The figure shows three views and two pictorial views of one solid part (mm, origin at its lowest corner). Answer the questions. Coordinates: 2 decimals unless noted, no trailing zeros. Order: outer loops, then holes, each group sorted by start corner. A loop starts at its lowest first (then second) coordinate and runs counter-clockwise, first axis right, second up. Notation, with made-up numbers: (17.25, 25) -> (72.25, 25) arc R20 cw to (72.25, 63) -> close; hole circle Ø2 at (75.5, 79). An arc over 180 degrees is marked (long way). Return JSON: item names as keys, results as strings.
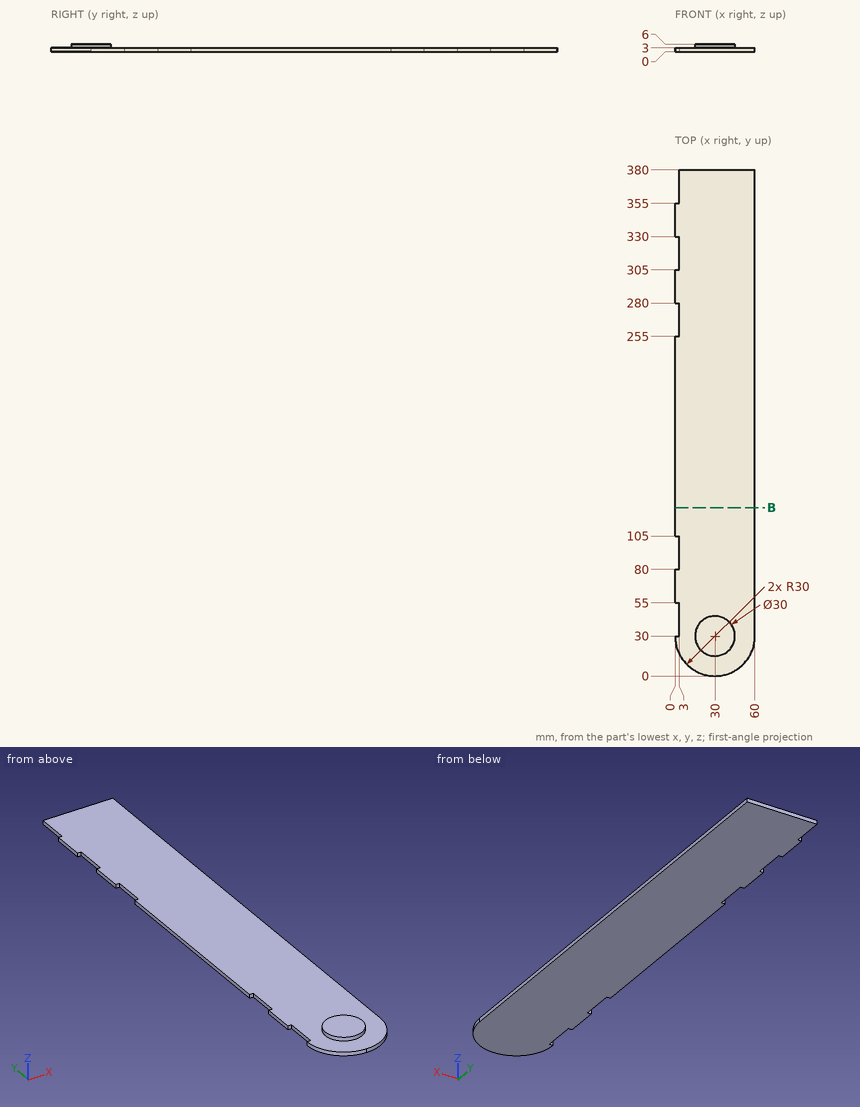
Item 1: Flat-ended cylindrical pins translate along their axes: pin 1 (0.9 mm diameter, centred on x = 1.5, z = 1, fed in from +Y); pin 2 (3.5 mm diameter, centred on x = 1.5, z = 1.5, fed in from -Y); pin 3 (6 mm diameter, centred on x = 23, y = 117, fed in from +Z). Find the tip coordinate at first contact, or state that the pin passes through.
Answer list:
{"pin 1": "y = 355", "pin 2": "y = 16.42", "pin 3": "z = 3"}
Item 2: Find the intervals of material crossed by probe 1 along Z at (x, y) = (4.5, 237); probe 2 along X at (y, z) = (358, 1.15); probe 3 along Y at (x, z) = (28.5, 5.7) (3 decimals), in increasing order.
Answer list:
{"probe 1": "0 to 3", "probe 2": "3 to 60", "probe 3": "15.075 to 44.925"}
Item 3: The part is cut by section B-B on y = 126.5. Determine the outline of the cut face in (x, z), plus the area to 3 significant figures.
Answer list:
{"outline": "(0, 0) -> (60, 0) -> (60, 3) -> (0, 3) -> close", "area": "180 mm2"}
